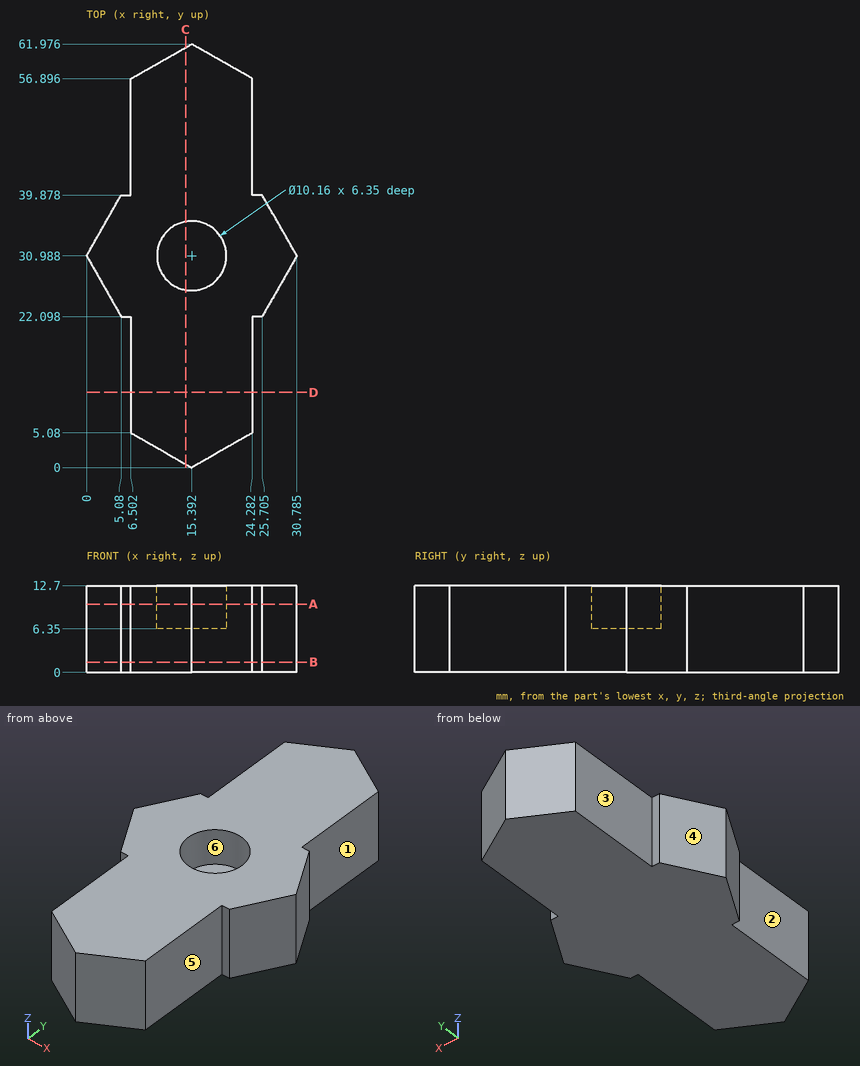
Answer from the drawing. Dimensions are ordinates in mm from the lowest x, y and z of the part. A direction names the side the tool comes from. Give positions to 0.01 mm unless a question says otherwise; leave off trailing zeros. Write each loop counter-clockwise with the first axis right and the second up, starting at its lowest first coordinate (ties: lowest second). Pieces come first, ordered by that corner, then holes. Notation, with made-up numbers: (53, 37) -> (111, 37) arc R8 cw to (111, 46) -> close; hole circle Ø9 at (52.5, 72.25). An arc over 180 degrees is marked (long way). One line per question, with ' | ' between items. Start each with the question number.
1. Section B-B (z = 1.5) is taken. Determine the outline of the cut face in (x, y) (1 decimal).
2. Find the intervals of material crossed by probe 1 along X at (y, z) = (10.5, 4.5); probe 2 along Z at (x, y) = (15.5, 34.5); probe 3 along Y at (x, z) = (15, 9.25) (1 decimal), in increasing order.
3. For the marked faces 1, 2 and 3, determine the directions among +Z, -Z, +X, -X, +Y, -Y from which every point of the face is accessible in a straight line to the end or side of a thin tool.
4. For a pull along X with two mould halves and no side action, classify the marked faces 4, 5 and 6 as pulls with the +X half, pulls with the -X half, needs draft (parallel to the pull), parting line crosses it, or undercut.
5. Section A-A (z = 10) is taken. Determine the outline of the cut face in (x, y) (1 decimal).
6. Section D-D (y = 11) is taken. Determine the outline of the cut face in (x, z).
7. Given pin 1 Ø6.5 at (y, z) = (45.5, 3) entering from -X; pin 2 Ø4 at (y, z) = (12.5, 6) entering from +X; pin 3 Ø1.6 at (x, z) = (6, 5) entering from -Y, each flat-ended and moving along its own axis, determine where each tip first touches the part or whether it passes through.
8. Section C-C (x = 14.5) is taken. Determine the outline of the cut face in (y, z).
Response values:
1) outline: (0, 31) -> (5.1, 22.1) -> (6.5, 22.1) -> (6.5, 5.1) -> (15.4, 0) -> (24.3, 5.1) -> (24.3, 22.1) -> (25.7, 22.1) -> (30.8, 31) -> (25.7, 39.9) -> (24.3, 39.9) -> (24.3, 56.9) -> (15.4, 62) -> (6.5, 56.9) -> (6.5, 39.9) -> (5.1, 39.9) -> close
2) probe 1: 6.5 to 24.28 | probe 2: 0 to 6.35 | probe 3: 0.2 to 25.9, 36.1 to 61.8
3) face 1: +Z, -Z, +X, +Y | face 2: +Z, -Z, -X, -Y | face 3: +Z, -Z, -X, +Y
4) face 4: pulls with the -X half | face 5: pulls with the +X half | face 6: undercut
5) outline: (0, 31) -> (5.1, 22.1) -> (6.5, 22.1) -> (6.5, 5.1) -> (15.4, 0) -> (24.3, 5.1) -> (24.3, 22.1) -> (25.7, 22.1) -> (30.8, 31) -> (25.7, 39.9) -> (24.3, 39.9) -> (24.3, 56.9) -> (15.4, 62) -> (6.5, 56.9) -> (6.5, 39.9) -> (5.1, 39.9) -> close; hole circle Ø10.2 at (15.4, 31)
6) outline: (6.5, 0) -> (24.28, 0) -> (24.28, 12.7) -> (6.5, 12.7) -> close
7) pin 1: x = 6.5 | pin 2: x = 24.28 | pin 3: y = 4.91
8) outline: (0.51, 0) -> (61.47, 0) -> (61.47, 12.7) -> (35.99, 12.7) -> (35.99, 6.35) -> (25.99, 6.35) -> (25.99, 12.7) -> (0.51, 12.7) -> close
